Here's how the part is built. I have some questions about the finished solid (model axes, mm). Face numbers are marked on the shaded views. Give positions to 0.01 mm unless a question says otherwise; leave off trailing zeros. Loops run counter-clockwise (first coordinate to the right, second up) from the corner with the lowest first, then second, coordinate; pieces in that order, holes last. Notation, with made-up numbers: (67.5, -19) - (71.5, -19) arc R31 ccw to (71.5, 14) - close; hole circle Ø2 at (-9.5, -30). An arc over 180 degrees is marked (long way). Use a Markdown table: item, result.
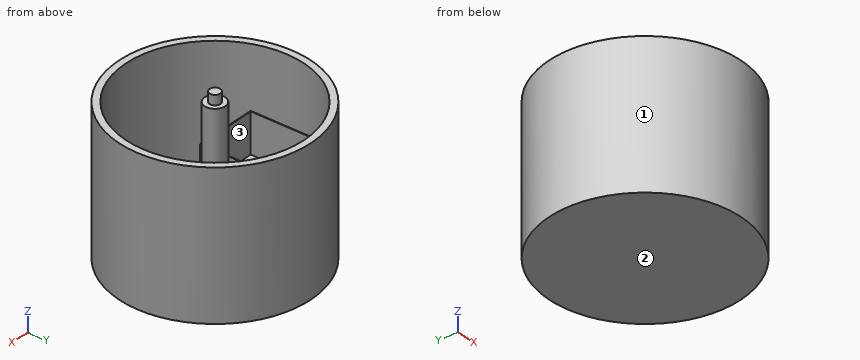
from build123d import *

# Parameters (mm, degrees)
SKETCH1_R                       = 69.53
SKETCH1_W                       = 42.3
SKETCH1_H                       = 42.3
BOSS_EXTRUDE1_DEPTH             = 104.14
SHELL1_T                        = -5
SKETCH1_4_W                     = 42.3
SKETCH1_4_H                     = 42.3
BOSS_EXTRUDE3_DEPTH             = 31.14
SKETCH2_W                       = 45.3
SKETCH2_H                       = 45.3
BOSS_EXTRUDE5_DEPTH             = 28.7
BOSS_EXTRUDE5_DIRECTION_2_REACH = 124.466
CUT_EXTRUDE1_START              = -28.7
SKETCH3_W                       = 44.3
SKETCH3_H                       = 44.3
CUT_EXTRUDE1_DEPTH              = 28.7
SKETCH4_R                       = 7.5
BOSS_EXTRUDE6_DEPTH             = 99.14
SKETCH5_R                       = 3.9
BOSS_EXTRUDE7_DEPTH             = 7


with BuildPart() as part:
    # Sketch1 → Boss-Extrude1 (new body)
    # profile 1 of 2: a face of its own
    with BuildSketch(Plane.XY):
        Circle(SKETCH1_R)
        with Locations((-37.305, 0)):
            Rectangle(SKETCH1_W, SKETCH1_H, mode=Mode.SUBTRACT)
    # profile 2 of 2: a face of its own
    with BuildSketch(Plane.XY):
        with Locations((-37.305, 0)):
            Rectangle(SKETCH1_W, SKETCH1_H)
    extrude(amount=BOSS_EXTRUDE1_DEPTH)

    # Shell1
    shell1_openings = [part.faces().sort_by_distance(p)[0] for p in [
        (0, 0, 104.14),
    ]]
    offset(amount=SHELL1_T, openings=shell1_openings, kind=Kind.INTERSECTION)

    # Sketch1<4> → Boss-Extrude3 (add)
    with BuildSketch(Plane.XY):
        with Locations((-37.305, 0)):
            Rectangle(SKETCH1_4_W, SKETCH1_4_H)
    extrude(amount=BOSS_EXTRUDE3_DEPTH)

    # Sketch2 → Boss-Extrude5 (add)
    with BuildSketch(Plane.XY.offset(31.14)):
        with Locations((-37.305, 0)):
            Rectangle(SKETCH2_W, SKETCH2_H)
        with BuildLine():
            Line((-58.455, -20.754129107), (-58.455, 20.754129107))
            ThreePointArc((-58.455, 20.754129107), (-58.384303073, 20.952184962), (-58.3129351, 21.15))
            Line((-58.3129351, 21.15), (-16.155, 21.15))
            Line((-16.155, 21.15), (-16.155, -21.15))
            Line((-16.155, -21.15), (-58.3129351, -21.15))
            ThreePointArc((-58.3129351, -21.15), (-58.384303073, -20.952184962), (-58.455, -20.754129107))
        make_face(mode=Mode.SUBTRACT)
    extrude(amount=BOSS_EXTRUDE5_DEPTH)

    # Sketch2 → Boss-Extrude5 direction 2 (add, up to next)
    with BuildSketch(Plane.XY.offset(31.14), mode=Mode.PRIVATE) as boss_extrude5_direction_2_sk1:
        with Locations((-37.305, 0)):
            Rectangle(SKETCH2_W, SKETCH2_H)
        with BuildLine():
            Line((-58.455, -20.754129107), (-58.455, 20.754129107))
            ThreePointArc((-58.455, 20.754129107), (-58.384303073, 20.952184962), (-58.3129351, 21.15))
            Line((-58.3129351, 21.15), (-16.155, 21.15))
            Line((-16.155, 21.15), (-16.155, -21.15))
            Line((-16.155, -21.15), (-58.3129351, -21.15))
            ThreePointArc((-58.3129351, -21.15), (-58.384303073, -20.952184962), (-58.455, -20.754129107))
        make_face(mode=Mode.SUBTRACT)
    boss_extrude5_direction_2_tool1 = extrude(boss_extrude5_direction_2_sk1.sketch, amount=-BOSS_EXTRUDE5_DIRECTION_2_REACH, mode=Mode.PRIVATE) - part.part
    add(boss_extrude5_direction_2_tool1.solids().sort_by_distance((-37.305, -22.009361, 31.14))[0])

    # Sketch3 → Cut-Extrude1 (cut)
    with BuildSketch(Plane.XY.offset(59.84).offset(CUT_EXTRUDE1_START)):
        with Locations((-37.305, 0)):
            Rectangle(SKETCH3_W, SKETCH3_H)
        with BuildLine():
            Line((-16.155, -21.15), (-58.3129351, -21.15))
            ThreePointArc((-58.3129351, -21.15), (-58.384303073, -20.952184962), (-58.455, -20.754129107))
            Line((-58.455, -20.754129107), (-58.455, 20.754129107))
            ThreePointArc((-58.455, 20.754129107), (-58.384303073, 20.952184962), (-58.3129351, 21.15))
            Line((-58.3129351, 21.15), (-16.155, 21.15))
            Line((-16.155, 21.15), (-16.155, -21.15))
        make_face(mode=Mode.SUBTRACT)
    extrude(amount=CUT_EXTRUDE1_DEPTH, mode=Mode.SUBTRACT)

    # Sketch4 → Boss-Extrude6 (add)
    with BuildSketch(Plane.XY.offset(5)):
        with Locations(Location((0, 0, 0), (0, 0, 180))):
            Circle(SKETCH4_R)
    extrude(amount=BOSS_EXTRUDE6_DEPTH)

    # Sketch5 → Boss-Extrude7 (add)
    with BuildSketch(Plane.XY.offset(104.14)):
        Circle(SKETCH5_R)
    extrude(amount=BOSS_EXTRUDE7_DEPTH)


solid = part.part
(1) Suppose I cut it at C-C on x = 0. Write out the boundary of the cut face in (y, z), plus the area to 3 significant figures.
A:
| item | result |
|---|---|
| outline | (-69.53, 0) - (69.53, 0) - (69.53, 104.14) - (64.53, 104.14) - (64.53, 5) - (7.5, 5) - (7.5, 104.14) - (3.9, 104.14) - (3.9, 111.14) - (-3.9, 111.14) - (-3.9, 104.14) - (-7.5, 104.14) - (-7.5, 5) - (-64.53, 5) - (-64.53, 104.14) - (-69.53, 104.14) - close |
| area | 3,230 mm2 |
(2) If I drill on line 1 (Y direction, x = 0, z = 80.5); line 2 (X direction, y = 6.5, z = 23) (1 decimal); line 3 (Y direction, x = -2.5, z = 26), over which ranges is the centre line in solid material (lowest first)?
A:
| item | result |
|---|---|
| line 1 | -69.53 to -64.53, -7.5 to 7.5, 64.53 to 69.53 |
| line 2 | -69.2 to -64.2, -60 to -14.7, -3.7 to 3.7, 64.2 to 69.2 |
| line 3 | -69.49 to -64.48, -7.07 to 7.07, 64.48 to 69.49 |
(3) Suppose I cut it at D-D on y = 0. Write out the boundary of the cut face in (x, z) (3 decimals), plus the area to 3 significant figures.
A:
| item | result |
|---|---|
| outline | (-69.53, 0) - (69.53, 0) - (69.53, 104.14) - (64.53, 104.14) - (64.53, 5) - (7.5, 5) - (7.5, 104.14) - (3.9, 104.14) - (3.9, 111.14) - (-3.9, 111.14) - (-3.9, 104.14) - (-7.5, 104.14) - (-7.5, 5) - (-14.655, 5) - (-14.655, 59.84) - (-15.155, 59.84) - (-15.155, 31.14) - (-59.455, 31.14) - (-59.455, 59.84) - (-59.955, 59.84) - (-59.955, 5) - (-64.53, 5) - (-64.53, 104.14) - (-69.53, 104.14) - close |
| area | 4,440 mm2 |
(4) We'd pull the mould along Y, two halves only. Please class the marked faces 1, 2 and 3: pulls with the +Y half, pulls with the -Y half, needs draft (parallel to the pull), parting line crosses it, or undercut.
A:
| item | result |
|---|---|
| face 1 | parting line crosses it |
| face 2 | needs draft |
| face 3 | undercut |
(5) Suppose I cut it at B-B on z = 65. Write out the boundary of the cut face in (x, y).
A:
| item | result |
|---|---|
| outline | circle Ø139.06 at (0, 0); circle Ø15 at (0, 0); hole circle Ø129.06 at (0, 0) |
(6) Suppose I cut it at A-A on z = 15.5. Write out the boundary of the cut face in (x, y) (3 decimals), plus the area to 3 significant figures.
A:
| item | result |
|---|---|
| outline | circle Ø139.06 at (0, 0); (-59.955, -22.65) - (-14.655, -22.65) - (-14.655, 22.65) - (-59.955, 22.65) - close; circle Ø15 at (0, 0); hole circle Ø129.06 at (0, 0) |
| area | 4,330 mm2 |
(7) Will these pins go through, and if not, where does the flat tip stop? pin 1 (22.5 mm diameter, centred on x = -45, z = 31, fed in from +Y); pin 2 (13.5 mm diameter, centred on x = -46, y = -7.5, fed in from +Z); pin 3 (1.5 mm diameter, centred on y = 20.5, z = 25.5, fed in from -X); pin 4 (12 mm diameter, centred on y = 3.5, z = 32.5, fed in from -X).
A:
| item | result |
|---|---|
| pin 1 | y = 60.79 |
| pin 2 | z = 31.14 |
| pin 3 | x = -66.67 |
| pin 4 | x = -69.53 |
